Autodesk Inventor part; units mm, degrees
ref_plane "YZ Plane" through (0, 0, 0) normal (1, 0, 0) x (0, 1, 0)
ref_plane "XZ Plane" through (0, 0, 0) normal (0, 1, 0) x (-1, 0, 0)
ref_plane "XY Plane" through (0, 0, 0) normal (0, 0, 1) x (1, 0, 0)
sketch "Sketch1" plane through (0, 0, 0) normal (0, 1, 0) x (-1, 0, 0)
  line L0 (-6.25, 18.75) -> (6.25, 18.75)
  line L1 (6.25, 18.75) -> (6.25, -18.75)
  line L2 (6.25, -18.75) -> (-6.25, -18.75)
  line L3 (-6.25, -18.75) -> (-6.25, 18.75)
  line L4 (5.25, 18.75) -> (5.25, -18.75)
  line L5 (-5.25, 18.75) -> (-5.25, -18.75)
  line L6 (5.25, 11.75) -> (-5.25, 11.75)
  line L7 (5.25, 5.75) -> (-5.25, 5.75)
  line L8 (5.25, -1.25) -> (-5.25, -1.25)
  line L9 (5.25, -9.25) -> (-5.25, -9.25)
  point P0 (0, 0)
  dimension "d0" = 12.5
  dimension "d1" = 37.5
extrude "Extrusion1" add sketch "Sketch1" along normal blind 1 contours L0 L5 L2 L3 | L0 L4 L6 L5 | L0 L1 L2 L4 | L5 L9 L4 L2 | L7 L4 L8 L5
properties part number "if_case_top"
Source: CAD feature listing. Evaluate the final solid. Frame: model axes, mm. A direction names the side the tool comes from. Coordinates: 2 decimals unless noted, no trailing zeros. Loops run counter-clockwise (first coordinate to the right, second up) from the corner with the lowest first, then second, coordinate; pieces in that order, holes last. Notation, with made-up numbers: M 14,48.25 L 30,48.25 A38 cw 30,87.25 Z; hole C -34,78 d2. An arc over 180 degrees is marked long. Use a Markdown table: item, result. Add a question column.
Q1. Access query for faces 5 (the flat face through (0.1, 0.5, 18.75)), 6 (the flat face through (5.25, 0.5, 8.8)). Directions: +Z, -Z, +X, -X, +Y, -Y. A direction counts if a zero-diameter tool reaches every point of the face in a straight line with its end or side. Return the directions, or none.
Q2. Draft query along X for faces 1 (the flat face through (6.25, 0.5, -0.3)), 2 (the flat face through (-5.25, 0.5, 8.8)), 3 (the flat face through (-5.25, 0.5, -5.2)), 4 (the flat face through (0, 1, 0)). Return one class per face: pulls with the +X half, pulls with the -X half, needs draft (parallel to the pull), parting line crosses it, or undercut.
Q3. Section query A-A, the plane x = 1.5. Return loops of the section in (y, z), and give its area (3 significant figures).
Q4. Material intervals for L1, parallel to Z at x = 0, y = 0.8; L2, parallel to X at y = 0.75, z = -8, sorted ascending.
Q5. Section query B-B, the plane y = 0.3. Return loops of the section in (x, z).
Result:
| question | item | result |
|---|---|---|
| 1 | face 5 | +Z, +X, -X, +Y, -Y |
| 1 | face 6 | +Y, -Y |
| 2 | face 1 | pulls with the +X half |
| 2 | face 2 | undercut |
| 2 | face 3 | undercut |
| 2 | face 4 | needs draft |
| 3 | outline | M 0,-18.75 L 1,-18.75 L 1,-9.25 L 0,-9.25 Z; M 0,-1.25 L 1,-1.25 L 1,5.75 L 0,5.75 Z; M 0,11.75 L 1,11.75 L 1,18.75 L 0,18.75 Z |
| 3 | area | 23.5 mm2 |
| 4 | L1 | z = -18.75 to -9.25, -1.25 to 5.75, 11.75 to 18.75 |
| 4 | L2 | x = -6.25 to -5.25, 5.25 to 6.25 |
| 5 | outline | M -6.25,-18.75 L 6.25,-18.75 L 6.25,18.75 L -6.25,18.75 Z; hole M -5.25,-9.25 L 5.25,-9.25 L 5.25,-1.25 L -5.25,-1.25 Z; hole M -5.25,5.75 L 5.25,5.75 L 5.25,11.75 L -5.25,11.75 Z |
